Autodesk Inventor part; units mm, degrees
ref_plane "YZ Plane" through (0, 0, 0) normal (1, 0, 0) x (0, 1, 0)
ref_plane "XZ Plane" through (0, 0, 0) normal (0, 1, 0) x (-1, 0, 0)
ref_plane "XY Plane" through (0, 0, 0) normal (0, 0, 1) x (1, 0, 0)
sketch "草图1" plane through (0, 0, 0) normal (0, 0, 1) x (1, 0, 0)
  circle A0 centre (0, 0) radius 6
  dimension "d0" = 12
extrude "拉伸1" add sketch "草图1" along normal blind 2
sketch "草图2" plane through (0, 0, 2) normal (0, 0, 1) x (1, 0, 0)
  circle A0 centre (0, 0) radius 6
  circle A1 centre (0, 0) radius 5.5
  dimension "d3" = 11
extrude "拉伸2" add sketch "草图2" along normal blind 2 contours A1
sketch "草图3" plane through (0, 0, 0) normal (0, 0, -1) x (-1, 0, 0)
  circle A0 centre (0, 0) radius 6
  circle A1 centre (0, 0) radius 3.75
  dimension "d6" = 7.5
extrude "拉伸3" add sketch "草图3" along normal blind 6 contours A1
sketch "草图4" plane through (0, 0, 0) normal (0, 1, 0) x (-1, 0, 0)
  line L0 (6, 2) -> (-6, 2)
  arc A0 (0, 14.4) -> (0, 2) centre (0, 8.2) ccw
  line L1 (0, 2) -> (0, 14.4)
  point P0 (0, 0)
revolve "旋转1" cut sketch "草图4" angle 360 about axis through (0, 0, 2) along (0, 0, 1)
chamfer "倒角1" distance 0.5 angle 45 4 edges at (3.75, 0, -6) (-6, 0, 0) (-6, 0, 2) (-5.5, 0, 4)
properties part number "钢珠定位圈" material "钢"
The model under review builds one solid part; all positions refer to its coordinate system, in mm. A direction names the side the tool comes from. Coordinates: 2 decimals unless noted, no trailing zeros. Write each loop counter-clockwise with the first axis right and the second up, starting at its lowest first coordinate (ties: lowest second). Pieces come first, ordered by that corner, then holes.
1) To check wall thickness, follow probe 1 along X at (y, z) = (-2, 3); probe 2 along Z at (x, y) = (1.75, -0.25); probe 3 along X at (y, z) = (0.25, -1.5). State the ranges of each line that lie inside material, in increasing order.
2) Clearance check with flat-ended pins moving along their axes: pin 1 Ø1.5 at (y, z) = (0.5, -0.5) entering from -X; pin 2 Ø1 at (x, y) = (4, 0) entering from -Z; pin 3 Ø5 at (x, y) = (-2.5, 4) entering from -Z. State where each tip first meets the part, or that it passes through.
3) Machinability: for faces 1 (the face through (-1.19, 5.37, 2.74)), 2 (the face through (0, 0, -6)), 3 (the face through (1, -4, 0)), which of the approach directions +Z, -Z, +X, -X, +Y, -Y give a long, thin tool a straight path to every point of the face, cutting with its end or side? Answer none if there is none.
4) We need section C-C on z = -0.25. State the section outline as (x, y) points, then the cut area to 3 significant figures.
5) We need section D-D on z = 3. State the section outline as (x, y) points.
Answer list:
1. probe 1: x = -5.12 to -2.72, 2.72 to 5.12
1. probe 2: z = -6 to 2.26
1. probe 3: x = -3.74 to 3.74
2. pin 1: stops at x = -5.73
2. pin 2: stops at z = -5.75
2. pin 3: stops at z = -6
3. face 1: +Z
3. face 2: -Z, +X, -X, +Y, -Y
3. face 3: -Z
4. outline: circle Ø7.5 at (0, 0)
4. area: 44.2 mm2
5. outline: circle Ø11 at (0, 0); hole circle Ø6.75 at (0, 0)
